Drawing for the job (mm, zero at the part's lowest x, y, z). Coordinates: 2 decimals unless noted, no trailing zeros. Write each loop counter-clockwise with the first axis right and the second up, starting at its lowest first coordinate (ties: lowest second). Pieces come first, ordered by that corner, then holes. Notation, with made-up numbers: (43, 31) - (77, 31) arc R30 cw to (77, 62) - close; hole circle Ø1 at (37, -26). An arc over 180 degrees is marked (long way). Write each question's results on one line, items separated by ' | '.
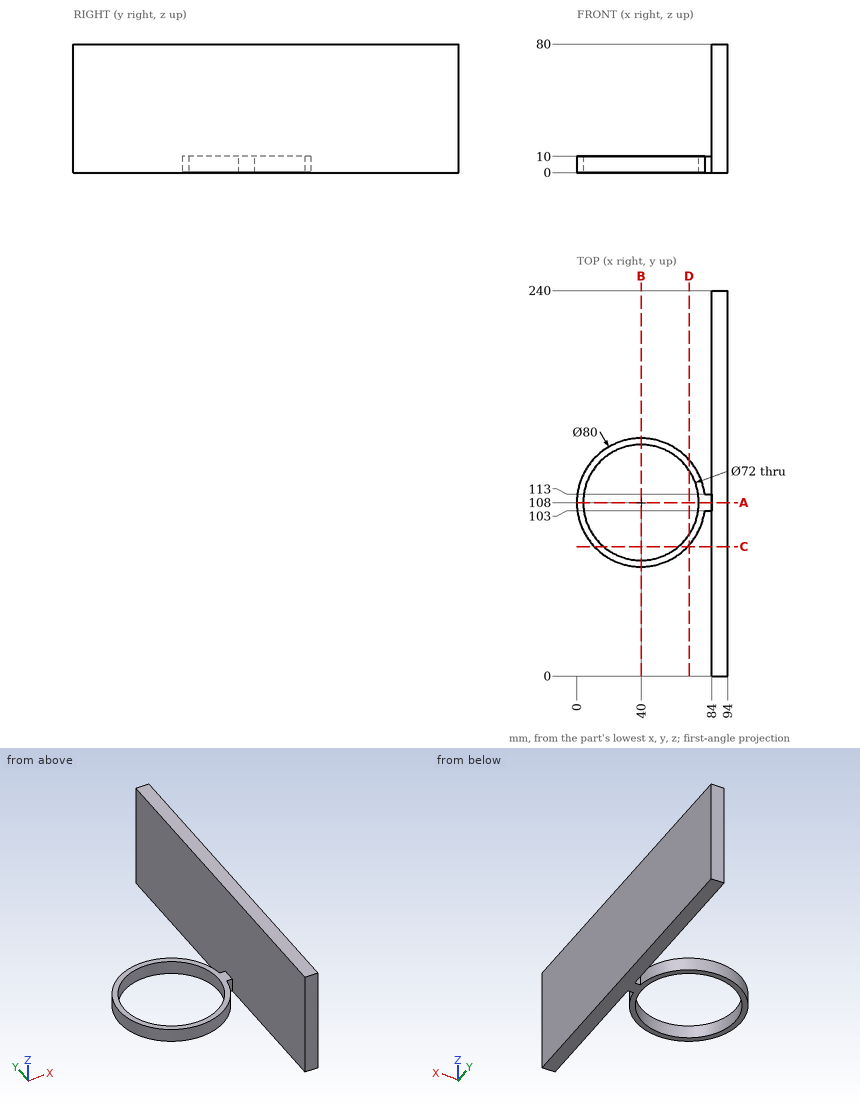
(1) Wall check: line 1 (Y direction, x = 40, z = 3); line 2 (X direction, y = 117.5, z = 33); line 3 (Z direction, x = 6, y = 129). Give the ranges that are in metal, low to high. Write a range as from..to.
Return value:
line 1: y = 68..72, 144..148 | line 2: x = 84..94 | line 3: z = 0..10
(2) Saw through at C-C on y = 80.5. Write the cut outline in (x, z).
Return value:
outline: (10.95, 0) - (16.77, 0) - (16.77, 10) - (10.95, 10) - close; (63.23, 0) - (69.05, 0) - (69.05, 10) - (63.23, 10) - close; (84, 0) - (94, 0) - (94, 80) - (84, 80) - close
(3) Flat gauge pins, fed straight in: P1, Ø1.3, axis at x = 82, z = 6.5, coming from the -Y side; P2, Ø1.3, axis at x = 82, z = 4.5, coming from the +Y side. Where does each tip first touch, or does it go through?
Return value:
P1: stops at y = 103 | P2: stops at y = 113
(4) Saw through at A-A on y = 108. Write the cut outline in (x, z).
Return value:
outline: (0, 0) - (4, 0) - (4, 10) - (0, 10) - close; (76, 0) - (94, 0) - (94, 80) - (84, 80) - (84, 10) - (76, 10) - close
(5) Saw through at B-B on x = 40. Write the cut outline in (y, z), then the cut area to 3 significant figures.
Return value:
outline: (68, 0) - (72, 0) - (72, 10) - (68, 10) - close; (144, 0) - (148, 0) - (148, 10) - (144, 10) - close | area: 80.0 mm^2
(6) Saw through at D-D on x = 70. Write the cut outline in (y, z), then the cut area to 3 significant figures.
Return value:
outline: (81.54, 0) - (88.1, 0) - (88.1, 10) - (81.54, 10) - close; (127.9, 0) - (134.46, 0) - (134.46, 10) - (127.9, 10) - close | area: 131 mm^2
